Geometry: final body of the model. Coordinates: model frame, mm. A direction names the side the tool comes from. Round coordinates to 2 decimals unless told otherwise and drop trailing zeros. Write each loop counter-clockwise with the first axis right and the second up, starting at its lowest first coordinate (ties: lowest second). Pieces come first, ordered by that corner, then holes. Notation, with made-up numbers: M 50.5,-39.75 L 101.5,-39.75 A26 ccw 101.5,-11.75 Z; hole C 44,86.5 d7. An arc over 180 degrees is marked long. Answer as CSV lines item,"result". Start each with the question number.
Q1. Section query D-D on x = 26. Give the number of separate pieces and of enclosed holes in the cut face, and give its area (3 significant figures).
Q2. Section query B-B on x = 37.5. Output: boundary loops of the cut face in (y, z), and give its area (3 significant figures).
Q3. First-contact query: pin 1 (3.5 mm diameter, centred on x = 5, z = 7, fed in from +Y); pin 2 (18 mm diameter, centred on x = 43.5, z = 56, fed in from -Y); pin 3 (7 mm diameter, centred on y = 12, z = 105.5, fed in from +X). Flat tips, straight axial feed; report the tip coordinate or a pass-through.
Q4. Ray query, probe 1 along X at (y, z) = (34.5, 8) (3 decimals); probe 2 along Z at (x, y) = (86.5, 25.5); probe 3 along X at (y, z) = (2, 57). Return the intervals inside material, ascending.
Q5. Section query A-A on y = 58.5. Output: boundary loops of the cut face in (x, z) (3 decimals), and give its area (3 significant figures).
Q6. Section query C-C on z = 29. Output: boundary loops of the cut face in (x, y) (3 decimals).
Q7. Reachability of faces 3 (the cylindrical face through (43.67, 1.48, 56.31)), 4 (the flat face through (49, 94.175, 90)), 5 (the flat face through (0.802, 81.143, 57.045)), 6 (the flat face through (1, 10, 10)) from +Z, -Z, +X, -X, +Y, -Y: full face, straight path, thin tool, end or side. Return the list, or none.
Q8. Mould query, pull axis X, two halves, no side actions, for faces 1 (the flat face through (50, 16, 3)), 2 (the flat face through (0.76, 87.077, 103.598)). Classes: pulls with the +X half, pulls with the -X half, needs draft (parallel to the pull), parting line crosses it, or undercut.
```python
from build123d import *

# Parameters (mm, degrees)
BOSS_EXTRUDE1_DEPTH = 100
SKETCH2_W           = 40
SKETCH2_H           = 3
BOSS_EXTRUDE2_DEPTH = 7.5
SKETCH3_W           = 60
SKETCH3_H           = 110
BOSS_EXTRUDE3_DEPTH = 3
BOSS_EXTRUDE4_DEPTH = 110
BOSS_EXTRUDE5_REACH = 183.953
SKETCH5_W           = 100
SKETCH5_H           = 2.5
CUT_EXTRUDE1_REACH  = 181.477
SKETCH6_R           = 1.5
SKETCH7_R           = 1.25
BOSS_EXTRUDE6_DEPTH = 2
CUT_EXTRUDE2_REACH  = 184.035
SKETCH8_R           = 1.75
SKETCH8_R_2         = 2.5
SKETCH8_W           = 78
SKETCH8_H           = 43.869493833
SKETCH8_W_2         = 27
SKETCH8_H_2         = 12
SKETCH9_W           = 87
SKETCH9_H           = 56
SKETCH9_W_2         = 30
SKETCH9_H_2         = 15
CUT_EXTRUDE3_DEPTH  = 2
SKETCH10_W          = 40
SKETCH10_H          = 20
CUT_EXTRUDE4_DEPTH  = 178.913626945
BOSS_EXTRUDE7_START = -1.5
SKETCH11_R          = 1.25
BOSS_EXTRUDE7_DEPTH = 1.5
CUT_EXTRUDE5_REACH  = 181.477


with BuildPart() as part:
    # Sketch1 → Boss-Extrude1 (new body)
    with BuildSketch(Plane(origin=(0, 0, 0), x_dir=(0, 0, -1), z_dir=(1, 0, 0))):
        Polygon((0, 0), (0, 30), (-67.175144213, 97.175144213), (-113, 97.175144213), (-113, 94.175144213), (-68.4177849, 94.175144213), (-3, 28.757359313), (-3, 0), align=None)
    extrude(amount=BOSS_EXTRUDE1_DEPTH)

    # Sketch2 → Boss-Extrude2 (add)
    with BuildSketch(Plane.XZ):
        with Locations((80, 1.5)):
            Rectangle(SKETCH2_W, SKETCH2_H)
    extrude(amount=BOSS_EXTRUDE2_DEPTH)

    # Sketch3 → Boss-Extrude3 (add)
    with BuildSketch(Plane.XZ):
        with Locations((30, 58)):
            Rectangle(SKETCH3_W, SKETCH3_H)
    extrude(amount=-BOSS_EXTRUDE3_DEPTH)

    # Sketch4 → Boss-Extrude4 (add)
    with BuildSketch(Plane.XY.offset(3)):
        Polygon((60, 3), (60, -7.5), (100, -7.5), (100, -5), (62.5, -5), (62.5, 3), align=None)
    extrude(amount=BOSS_EXTRUDE4_DEPTH)

    # Sketch5 → Boss-Extrude5 (add, up to next)
    with BuildSketch(Plane.XZ.offset(-94.175144213), mode=Mode.PRIVATE) as boss_extrude5_sk1:
        with Locations((50, 111.75)):
            Rectangle(SKETCH5_W, SKETCH5_H)
    boss_extrude5_tool1 = extrude(boss_extrude5_sk1.sketch, amount=BOSS_EXTRUDE5_REACH, mode=Mode.PRIVATE) - part.part
    add(boss_extrude5_tool1.solids().sort_by_distance((50, 94.175144, 111.75))[0])

    # Sketch6 → Cut-Extrude1 (cut, up to next)
    with BuildSketch(Plane.XZ, mode=Mode.PRIVATE) as cut_extrude1_sk1:
        with Locations(Location((5, 107, 0), (0, 0, 270))):
            Circle(SKETCH6_R)
    cut_extrude1_tool1 = extrude(cut_extrude1_sk1.sketch, amount=-CUT_EXTRUDE1_REACH, mode=Mode.PRIVATE) & part.part
    # Sketch6 → Cut-Extrude1 (cut, up to next)
    with BuildSketch(Plane.XZ, mode=Mode.PRIVATE) as cut_extrude1_sk2:
        with Locations(Location((45, 107, 0), (0, 0, 270))):
            Circle(SKETCH6_R)
    cut_extrude1_tool2 = extrude(cut_extrude1_sk2.sketch, amount=-CUT_EXTRUDE1_REACH, mode=Mode.PRIVATE) & part.part
    # Sketch6 → Cut-Extrude1 (cut, up to next)
    with BuildSketch(Plane.XZ, mode=Mode.PRIVATE) as cut_extrude1_sk3:
        with Locations(Location((45, 57, 0), (0, 0, 270))):
            Circle(SKETCH6_R)
    cut_extrude1_tool3 = extrude(cut_extrude1_sk3.sketch, amount=-CUT_EXTRUDE1_REACH, mode=Mode.PRIVATE) & part.part
    # Sketch6 → Cut-Extrude1 (cut, up to next)
    with BuildSketch(Plane.XZ, mode=Mode.PRIVATE) as cut_extrude1_sk4:
        with Locations(Location((5, 57, 0), (0, 0, 270))):
            Circle(SKETCH6_R)
    cut_extrude1_tool4 = extrude(cut_extrude1_sk4.sketch, amount=-CUT_EXTRUDE1_REACH, mode=Mode.PRIVATE) & part.part
    # Sketch6 → Cut-Extrude1 (cut, up to next)
    with BuildSketch(Plane.XZ, mode=Mode.PRIVATE) as cut_extrude1_sk5:
        with Locations(Location((5, 7, 0), (0, 0, 270))):
            Circle(SKETCH6_R)
    cut_extrude1_tool5 = extrude(cut_extrude1_sk5.sketch, amount=-CUT_EXTRUDE1_REACH, mode=Mode.PRIVATE) & part.part
    # Sketch6 → Cut-Extrude1 (cut, up to next)
    with BuildSketch(Plane.XZ, mode=Mode.PRIVATE) as cut_extrude1_sk6:
        with Locations(Location((45, 7, 0), (0, 0, 270))):
            Circle(SKETCH6_R)
    cut_extrude1_tool6 = extrude(cut_extrude1_sk6.sketch, amount=-CUT_EXTRUDE1_REACH, mode=Mode.PRIVATE) & part.part
    add(cut_extrude1_tool1.solids().sort_by_distance((5, 0, 107))[0], mode=Mode.SUBTRACT)
    add(cut_extrude1_tool2.solids().sort_by_distance((45, 0, 107))[0], mode=Mode.SUBTRACT)
    add(cut_extrude1_tool3.solids().sort_by_distance((45, 0, 57))[0], mode=Mode.SUBTRACT)
    add(cut_extrude1_tool4.solids().sort_by_distance((5, 0, 57))[0], mode=Mode.SUBTRACT)
    add(cut_extrude1_tool5.solids().sort_by_distance((5, 0, 7))[0], mode=Mode.SUBTRACT)
    add(cut_extrude1_tool6.solids().sort_by_distance((45, 0, 7))[0], mode=Mode.SUBTRACT)

    # Sketch7 → Boss-Extrude6 (add)
    # profile 1 of 4: a face of its own
    with BuildSketch(Plane(origin=(100, 0, 0), x_dir=(0, 0, -1), z_dir=(1, 0, 0))):
        Polygon((-110.5, -5), (-110.5, 9), (-96.5, -5), align=None)
        with Locations((-107, -1.5)):
            Circle(SKETCH7_R, mode=Mode.SUBTRACT)
    # profile 2 of 4: a face of its own
    with BuildSketch(Plane(origin=(100, 0, 0), x_dir=(0, 0, -1), z_dir=(1, 0, 0))):
        Polygon((-110.5, 94.175144213), (-110.5, 80.175144213), (-96.5, 94.175144213), align=None)
        with Locations((-107, 90.675144213)):
            Circle(SKETCH7_R, mode=Mode.SUBTRACT)
    # profile 3 of 4: a face of its own
    with BuildSketch(Plane(origin=(100, 0, 0), x_dir=(0, 0, -1), z_dir=(1, 0, 0))):
        Polygon((-82.4177849, 94.175144213), (-3, 14.757359313), (-3, 28.757359313), (-68.4177849, 94.175144213), align=None)
        with Locations((-6.5, 25.257359313)):
            Circle(SKETCH7_R, mode=Mode.SUBTRACT)
        with Locations((-71.9177849, 90.675144213)):
            Circle(SKETCH7_R, mode=Mode.SUBTRACT)
    # profile 4 of 4: a face of its own
    with BuildSketch(Plane(origin=(100, 0, 0), x_dir=(0, 0, -1), z_dir=(1, 0, 0))):
        Polygon((-17, -5), (-3, 9), (-3, -5), align=None)
        with Locations((-6.5, -1.5)):
            Circle(SKETCH7_R, mode=Mode.SUBTRACT)
    extrude(amount=-BOSS_EXTRUDE6_DEPTH)

    # Sketch8 → Cut-Extrude2 (cut, up to next)
    with BuildSketch(Plane(origin=(0, 15, -15), x_dir=(1, 0, 0), z_dir=(0, 0.7071067811865488, -0.7071067811865464)), mode=Mode.PRIVATE) as cut_extrude2_sk1:
        with Locations(Location((6.05, -109.488203436, 0), (0, 0, 270))):
            Circle(SKETCH8_R)
    cut_extrude2_tool1 = extrude(cut_extrude2_sk1.sketch, amount=-CUT_EXTRUDE2_REACH, mode=Mode.PRIVATE) & part.part
    # Sketch8 → Cut-Extrude2 (cut, up to next)
    with BuildSketch(Plane(origin=(0, 15, -15), x_dir=(1, 0, 0), z_dir=(0, 0.7071067811865488, -0.7071067811865464)), mode=Mode.PRIVATE) as cut_extrude2_sk2:
        with Locations(Location((93.95, -109.488203436, 0), (0, 0, 270))):
            Circle(SKETCH8_R)
    cut_extrude2_tool2 = extrude(cut_extrude2_sk2.sketch, amount=-CUT_EXTRUDE2_REACH, mode=Mode.PRIVATE) & part.part
    # Sketch8 → Cut-Extrude2 (cut, up to next)
    with BuildSketch(Plane(origin=(0, 15, -15), x_dir=(1, 0, 0), z_dir=(0, 0.7071067811865488, -0.7071067811865464)), mode=Mode.PRIVATE) as cut_extrude2_sk3:
        with Locations(Location((93.95, -44.588203436, 0), (0, 0, 270))):
            Circle(SKETCH8_R)
    cut_extrude2_tool3 = extrude(cut_extrude2_sk3.sketch, amount=-CUT_EXTRUDE2_REACH, mode=Mode.PRIVATE) & part.part
    # Sketch8 → Cut-Extrude2 (cut, up to next)
    with BuildSketch(Plane(origin=(0, 15, -15), x_dir=(1, 0, 0), z_dir=(0, 0.7071067811865488, -0.7071067811865464)), mode=Mode.PRIVATE) as cut_extrude2_sk4:
        with Locations(Location((6.05, -44.588203436, 0), (0, 0, 270))):
            Circle(SKETCH8_R)
    cut_extrude2_tool4 = extrude(cut_extrude2_sk4.sketch, amount=-CUT_EXTRUDE2_REACH, mode=Mode.PRIVATE) & part.part
    # Sketch8 → Cut-Extrude2 (cut, up to next)
    with BuildSketch(Plane(origin=(0, 15, -15), x_dir=(1, 0, 0), z_dir=(0, 0.7071067811865488, -0.7071067811865464)), mode=Mode.PRIVATE) as cut_extrude2_sk5:
        with Locations(Location((51.495, -33.713203436, 0), (0, 0, 270))):
            Circle(SKETCH8_R_2)
    cut_extrude2_tool5 = extrude(cut_extrude2_sk5.sketch, amount=-CUT_EXTRUDE2_REACH, mode=Mode.PRIVATE) & part.part
    # Sketch8 → Cut-Extrude2 (cut, up to next)
    with BuildSketch(Plane(origin=(0, 15, -15), x_dir=(1, 0, 0), z_dir=(0, 0.7071067811865488, -0.7071067811865464)), mode=Mode.PRIVATE) as cut_extrude2_sk6:
        with Locations((50.025, -80.778456519)):
            Rectangle(SKETCH8_W, SKETCH8_H)
    cut_extrude2_tool6 = extrude(cut_extrude2_sk6.sketch, amount=-CUT_EXTRUDE2_REACH, mode=Mode.PRIVATE) & part.part
    # Sketch8 → Cut-Extrude2 (cut, up to next)
    with BuildSketch(Plane(origin=(0, 15, -15), x_dir=(1, 0, 0), z_dir=(0, 0.7071067811865488, -0.7071067811865464)), mode=Mode.PRIVATE) as cut_extrude2_sk7:
        with Locations((19.675, -34.213203436)):
            Rectangle(SKETCH8_W_2, SKETCH8_H_2)
    cut_extrude2_tool7 = extrude(cut_extrude2_sk7.sketch, amount=-CUT_EXTRUDE2_REACH, mode=Mode.PRIVATE) & part.part
    add(cut_extrude2_tool1.solids().sort_by_distance((6.05, 92.419851, 62.419851))[0], mode=Mode.SUBTRACT)
    add(cut_extrude2_tool2.solids().sort_by_distance((93.95, 92.419851, 62.419851))[0], mode=Mode.SUBTRACT)
    add(cut_extrude2_tool3.solids().sort_by_distance((93.95, 46.528621, 16.528621))[0], mode=Mode.SUBTRACT)
    add(cut_extrude2_tool4.solids().sort_by_distance((6.05, 46.528621, 16.528621))[0], mode=Mode.SUBTRACT)
    add(cut_extrude2_tool5.solids().sort_by_distance((51.495, 38.838835, 8.838835))[0], mode=Mode.SUBTRACT)
    add(cut_extrude2_tool6.solids().sort_by_distance((50.025, 72.118994, 42.118994))[0], mode=Mode.SUBTRACT)
    add(cut_extrude2_tool7.solids().sort_by_distance((19.675, 39.192388, 9.192388))[0], mode=Mode.SUBTRACT)

    # Sketch9 → Cut-Extrude3 (cut)
    with BuildSketch(Plane(origin=(0, 12.878679656, -12.878679656), x_dir=(1, 0, 0), z_dir=(0, -0.7071067811865489, 0.7071067811865461))):
        with Locations((48.525, 77.713203436)):
            Rectangle(SKETCH9_W, SKETCH9_H)
        with Locations((19.675, 34.213203436)):
            Rectangle(SKETCH9_W_2, SKETCH9_H_2)
    extrude(amount=-CUT_EXTRUDE3_DEPTH, mode=Mode.SUBTRACT)

    # Sketch10 → Cut-Extrude4 (cut, through all)
    with BuildSketch(Plane(origin=(0, 0, 110.5), x_dir=(-1, 0, 0), z_dir=(0, 0, -1))):
        with Locations((-25, 16)):
            Rectangle(SKETCH10_W, SKETCH10_H)
    extrude(amount=-CUT_EXTRUDE4_DEPTH, mode=Mode.SUBTRACT)

    # Sketch11 → Boss-Extrude7 (add)
    # profile 1 of 3: a face of its own
    with BuildSketch(Plane.ZY.offset(BOSS_EXTRUDE7_START)):
        Polygon((110.5, 94.175144213), (110.5, 80.175144213), (96.5, 94.175144213), align=None)
        with Locations(Location((107, 90.675144213, 0), (0, 0, 180))):
            Circle(SKETCH11_R, mode=Mode.SUBTRACT)
    # profile 2 of 3: a face of its own
    with BuildSketch(Plane.ZY.offset(BOSS_EXTRUDE7_START)):
        Polygon((68.4177849, 94.175144213), (82.4177849, 94.175144213), (4.121320344, 15.878679656), (17, 3), (3, 3), (3, 14.757359313), (3, 28.757359313), align=None)
        with Locations(Location((71.9177849, 90.675144213, 0), (0, 0, 180))):
            Circle(SKETCH11_R, mode=Mode.SUBTRACT)
        with Locations(Location((6.5, 25.257359313, 0), (0, 0, 180))):
            Circle(SKETCH11_R, mode=Mode.SUBTRACT)
        with Locations((6.5, 6.5)):
            Circle(SKETCH11_R, mode=Mode.SUBTRACT)
    # profile 3 of 3: a face of its own
    with BuildSketch(Plane.ZY.offset(BOSS_EXTRUDE7_START)):
        Polygon((96.5, 3), (110.5, 17), (110.5, 3), align=None)
        with Locations((107, 6.5)):
            Circle(SKETCH11_R, mode=Mode.SUBTRACT)
    extrude(amount=BOSS_EXTRUDE7_DEPTH)

    # Sketch12 → Cut-Extrude5 (cut, up to next)
    with BuildSketch(Plane.ZY, mode=Mode.PRIVATE) as cut_extrude5_sk1:
        Polygon((21.213203436, 49.091883092), (55.154328933, 83.033008589), (60.104076401, 78.083261121), (26.162950904, 44.142135624), align=None)
    cut_extrude5_tool1 = extrude(cut_extrude5_sk1.sketch, amount=-CUT_EXTRUDE5_REACH, mode=Mode.PRIVATE) & part.part
    add(cut_extrude5_tool1.solids().sort_by_distance((0, 63.587572, 40.65864))[0], mode=Mode.SUBTRACT)


solid = part.part
```
Entries:
1,separate pieces,"3"
1,enclosed holes,"0"
1,area,"815 mm^2"
2,outline,"M 0,0 L 30,0 L 56.61,26.61 L 55.9,27.32 L 49.45,20.86 L 48.03,22.27 L 28.76,3 L 3,3 L 3,110.5 L 6,110.5 L 6,113 L 0,113 Z; M 26,110.5 L 94.18,110.5 L 94.18,68.42 L 87.63,61.87 L 89.04,60.46 L 86.92,58.34 L 87.63,57.63 L 97.18,67.18 L 97.18,113 L 26,113 Z"
2,area,"857 mm^2"
3,pin 1,"stops at y = 38.75"
3,pin 2,"stops at y = 0"
3,pin 3,"stops at x = 1.5"
4,probe 1,"x = 0 to 4.675, 34.675 to 100"
4,probe 2,"z = 0 to 3, 110.5 to 113"
4,probe 3,"x = 0 to 3.5, 6.5 to 43.5, 46.5 to 62.5"
5,outline,"M 0,28.5 L 11.025,28.5 L 11.025,29.914 L 5.025,29.914 L 5.025,30.621 L 0,30.621 Z; M 0,40.521 L 1.5,40.521 L 1.5,46.743 L 0,46.743 Z; M 0,110.5 L 100,110.5 L 100,113 L 0,113 Z; M 89.025,28.5 L 100,28.5 L 100,46.743 L 98,46.743 L 98,32.743 L 92.025,32.743 L 92.025,29.914 L 89.025,29.914 Z"
5,area,"345 mm^2"
6,outline,"M 0,0 L 60,0 L 60,-7.5 L 100,-7.5 L 100,-5 L 62.5,-5 L 62.5,3 L 0,3 Z; M 0,40.757 L 1.5,40.757 L 1.5,46.979 L 0,46.979 Z; M 0,56.879 L 5.025,56.879 L 5.025,57.586 L 11.025,57.586 L 11.025,59 L 0,59 Z; M 89.025,57.586 L 92.025,57.586 L 92.025,54.757 L 98,54.757 L 98,40.757 L 100,40.757 L 100,59 L 89.025,59 Z"
7,face 3,"-Y"
7,face 4,"none"
7,face 5,"-X"
7,face 6,"+X, -X"
8,face 1,"undercut"
8,face 2,"needs draft"
